Read the model definition and answer for the solid it produces. Units are mm, in the model's axes. Face numbers are marked on the shaded views. A direction names the side the tool comes from. Coordinates: 2 decimals unless noted, no trailing zeros. Order: outer loops, then holes, each group sorted by start corner. A loop starts at its lowest first (then second) coordinate and runs counter-clockwise, first axis right, second up. Notation, with made-up numbers: (1.25, -19) - (21.25, -19) arc R17 ccw to (21.25, 8) - close; hole circle Ø10 at (-16.75, 50). An arc over 180 degrees is marked (long way). Use one line per item in the form item = value. Start each with the question number.
Autodesk Inventor part; units mm, degrees
ref_plane "YZ Plane" through (0, 0, 0) normal (1, 0, 0) x (0, 1, 0)
ref_plane "XZ Plane" through (0, 0, 0) normal (0, 1, 0) x (-1, 0, 0)
ref_plane "XY Plane" through (0, 0, 0) normal (0, 0, 1) x (1, 0, 0)
sketch "Sketch1" plane through (0, 0, 0) normal (0, 0, 1) x (1, 0, 0)
  line L0 (0, 72) -> (-10, 72)
  line L1 (-10, 72) -> (-10, 10)
  line L2 (-10, 10) -> (-40, 10)
  line L3 (-40, 10) -> (-40, 0)
  line L4 (-40, 0) -> (0, 0)
  line L5 (0, 0) -> (0, 72)
  dimension "d0" = 10
  dimension "d1" = 40
  dimension "d2" = 10
  dimension "d3" = 72
extrude "Extrusion1" add sketch "Sketch1" along normal mid plane 20
sketch "Sketch2" plane through (0, 0, 10) normal (1, 0, 0) x (0, 0, -1)
  circle A0 centre (10, 60) radius 7
  line L0 (20, 72) -> (0, 72)
  point P0 (10, 0)
  dimension "d6" = 0
  dimension "d7" = 12
  dimension "d8" = 14
extrude "Extrusion2" cut sketch "Sketch2" against normal up to surface (10 mm away)
fillet "Fillet1" radius 4 3 edges at (-5, 72, 10) (-5, 72, -10) (-10, 10, 0)
sketch "Sketch3" plane through (-40, 10, 10) normal (0, 1, 0) x (1, 0, 0)
  line L0 (26, 0) -> (0, 0)
  line L1 (0, 20) -> (26, 20)
  line L2 (0, 20) -> (0, 0)
  point P0 (40, 10)
  point P1 (7, 10)
  point P2 (20, 10)
  dimension "d19" = 20
  dimension "d20" = 10
  dimension "d21" = 0
  dimension "d22" = 7
  dimension "d23" = 13
hole "Hole1" at (-33, 10, 0) at (-20, 10, 0) direction (0, -1, 0) diameter 5.5 depth 10 counterbore diameter 9 counterbore depth 5
properties part number "induction_adapter" material "ABS Plastic"
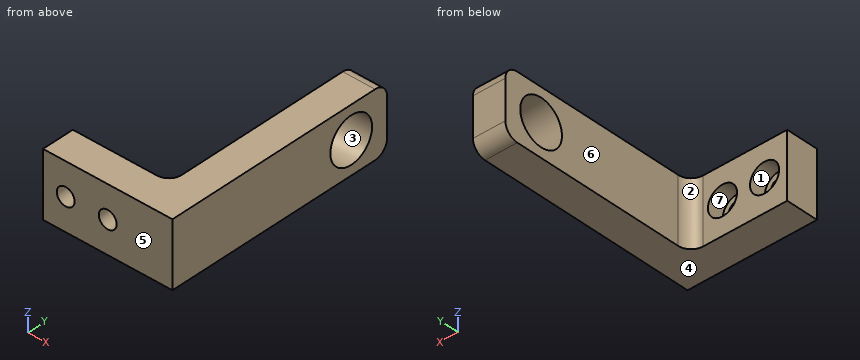
Q1. A cutting plane is placed at A-A (y = 60). Give the vertices of the cut face in (x, z).
Q2. For a pull along Z with two mould halves and no side action, classify the marked faces 1, 2, 3 and 4 as +Z half, -Z half, draft (parallel to the pull), parting line (faces both ways), or undercut.
Q3. Given P1, Ø6, axis at x = -27, y = 14, coming from the +Z side; P2, Ø4, axis at y = 45, z = 4, coming from the -X side; P3, Ø10, axis at x = -22, z = 0.5, coming from the +Y side, each flat-ended and moving along its own axis, determine where each tip first touches the part or whether it passes through.
Q4. A cutting plane is placed at C-C (z = 0). Give the vertices of the cut face in (x, y).
Q5. A cutting plane is placed at B-B (x = -20). Give the vertices of the cut face in (y, z).
Q6. A cutting plane is placed at D-D (x = -5). Give the vertices of the cut face in (y, z), then the cut area to 3 significant figures.
Q7. Consider probe 1 along X at (y, z) = (8.95, 0); probe 2 along X at (y, z) = (1.45, 0); probe 3 along Z at (x, y) = (-20, 3). Determine where each line is inside the solid, lowest interval first.
Q8. Which of the six approach directions +Z, -Z, +X, -X, +Y, -Y give full straight-line access (tool end or side, diameter ignored) to the marked faces 5, 6 and 7?
Result sheet:
q1.outline = (-10, -10) - (0, -10) - (0, -7) - (-10, -7) - close; (-10, 7) - (0, 7) - (0, 10) - (-10, 10) - close
q2.face_1 = undercut
q2.face_2 = draft
q2.face_3 = undercut
q2.face_4 = -Z half
q3.P1 = through
q3.P2 = -10
q3.P3 = 10
q4.outline = (-40, 0) - (-35.75, 0) - (-35.75, 5) - (-37.5, 5) - (-37.5, 10) - (-40, 10) - close; (-30.25, 0) - (-22.75, 0) - (-22.75, 5) - (-24.5, 5) - (-24.5, 10) - (-28.5, 10) - (-28.5, 5) - (-30.25, 5) - close; (-17.25, 0) - (0, 0) - (0, 53) - (-10, 53) - (-10, 14) arc R4 cw to (-14, 10) - (-15.5, 10) - (-15.5, 5) - (-17.25, 5) - close; (-10, 67) - (0, 67) - (0, 72) - (-10, 72) - close
q5.outline = (0, -10) - (10, -10) - (10, -4.5) - (5, -4.5) - (5, -2.75) - (0, -2.75) - close; (0, 2.75) - (5, 2.75) - (5, 4.5) - (10, 4.5) - (10, 10) - (0, 10) - close
q6.outline = (0, -10) - (68, -10) arc R4 ccw to (72, -6) - (72, 6) arc R4 ccw to (68, 10) - (0, 10) - close; hole circle Ø14 at (60, 0)
q6.area = 1,280 mm^2
q7.probe_1 = -40 to -37.5, -28.5 to -24.5, -15.5 to 0
q7.probe_2 = -40 to -35.75, -30.25 to -22.75, -17.25 to 0
q7.probe_3 = -10 to -2.75, 2.75 to 10
q8.face_5 = +Z, -Z, +X, -X, -Y
q8.face_6 = +Z, -Z, -X, +Y
q8.face_7 = +Y
